```python
from build123d import *

# Parameters (mm, degrees)
IZIM1_R                     = 1.5
Y_KSEKLIK_EKSTR_ZYON1_DEPTH = 50
IZIM2_W                     = 4.324361658
IZIM2_H                     = 3.770180851
KES_EKSTR_ZYON1_DEPTH       = 50


with BuildPart() as part:
    # Çizim1 → Yükseklik-Ekstrüzyon1 (new body)
    with BuildSketch(Plane.XY):
        with BuildLine():
            Line((0, 0), (-24.748737342, -24.748737342))
            ThreePointArc((-24.748737342, -24.748737342), (-9.324883978, -33.734945365), (8.524559631, -33.946014245))
            Line((8.524559631, -33.946014245), (0, 0))
        make_face()
        with Locations((-5.054296408, -19.108631106)):
            Circle(IZIM1_R, mode=Mode.SUBTRACT)
    extrude(amount=Y_KSEKLIK_EKSTR_ZYON1_DEPTH)

    # Çizim2 → Kes-Ekstrüzyon1 (cut)
    with BuildSketch(Plane.XY.offset(50)):
        with Locations((-5.054296408, -19.108631106)):
            Rectangle(IZIM2_W, IZIM2_H)
    extrude(amount=-KES_EKSTR_ZYON1_DEPTH, mode=Mode.SUBTRACT)


solid = part.part
```
Input: part model. Units: mm. Frame: model coordinates. A direction names the side the tool comes from. Round coordinates to 2 decimals unless told otherwise and drop trailing zeros. Write each loop counter-clockwise with the first axis right and the second up, starting at its lowest first coordinate (ties: lowest second). Pieces come first, ordered by that corner, then holes. Notation, with made-up numbers: (14, 50) -> (33, 50) arc R19 ccw to (33, 69) -> close; hole circle Ø8 at (9.5, -8.75). An arc over 180 degrees is marked (long way). Answer as CSV lines item,"result".
1. Reachability of faces 4 (the flat face through (-4.648, -21.144, 0)), 5 (the flat face through (-2.892, -19, 25)) from +Z, -Z, +X, -X, +Y, -Y: full face, straight path, thin tool, end or side. Return the list, or none.
Geometry says:
face 4,"-Z, +X, -X, +Y, -Y"
face 5,"+Z, -Z"
2. Mould query, pull axis Y, two halves, no side actions, for faces 1 (the flat face through (-4.648, -21.144, 50)), 2 (the flat face through (-5, -20.994, 25)), 3 (the cylindrical face through (-9.568, -33.667, 24.65)). Classes: +Y half, -Y half, draft (parallel to the pull), parting line (faces both ways), or undercut.
Geometry says:
face 1,"draft"
face 2,"undercut"
face 3,"-Y half"
3. Section B-B (y = -18.5). Return the cut outline in (x, z), plus the area to 3 significant figures.
Geometry says:
outline,"(-18.5, 0) -> (-7.22, 0) -> (-7.22, 50) -> (-18.5, 50) -> close; (-2.89, 0) -> (4.65, 0) -> (4.65, 50) -> (-2.89, 50) -> close"
area,"941 mm^2"
4. Section A-A (z = 46). Return the cut outline in (x, y), plus the area to 3 significant figures.
Geometry says:
outline,"(-24.75, -24.75) arc R35 ccw to (8.52, -33.95) -> (0, 0) -> close; hole (-7.22, -20.99) -> (-2.89, -20.99) -> (-2.89, -17.22) -> (-7.22, -17.22) -> close"
area,"615 mm^2"
5. Section C-C (x = -19). Return the cut outline in (y, z), plus the area to 3 significant figures.
Geometry says:
outline,"(-29.39, 0) -> (-19, 0) -> (-19, 50) -> (-29.39, 50) -> close"
area,"520 mm^2"
6. Ray query, L1, parallel to Y at x = -7, z = 37; L2, parallel to X at y = -20, z = 29.5; L3, parallel to Y at x = -6.5, z = 15.5. Return the intervals inside material, ascending. Write a range as [from, to].
Geometry says:
L1,"y = [-34.29, -20.99], [-17.22, -7]"
L2,"x = [-20, -7.22], [-2.89, 5.02]"
L3,"y = [-34.39, -20.99], [-17.22, -6.5]"
7. Contact query for flat-ended pins moving along their axis: P1, Ø1.5, axis at x = -8.5, z = 33.5, coming from the -Y side; P2, Ø3.5, axis at x = -4.5, z = 28, coming from the -Y side; P3, Ø4, axis at y = -19.5, z = 29.5, coming from the +X side; P4, Ø8, axis at x = -15, y = -7, coming from the -Z side. Output: stop coordinate, or through.
Geometry says:
P1,"stops at y = -34.13"
P2,"stops at y = -34.89"
P3,"stops at x = 5.4"
P4,"passes through"
8. Section D-D (y = -24). Return the cut outline in (x, z).
Geometry says:
outline,"(-24, 0) -> (6.03, 0) -> (6.03, 50) -> (-24, 50) -> close"
